from build123d import *

# Parameters (mm, degrees)
SKETCH_1_W      = 88
SKETCH_1_H      = 80
SKETCH_1_R      = 3
EXTRUDE_1_DEPTH = 3


with BuildPart() as part:
    # 草图1 → 凸台-拉伸1 (new body)
    with BuildSketch(Plane.XY):
        with Locations((-6, 0)):
            Rectangle(SKETCH_1_W, SKETCH_1_H)
        with Locations((-27, 25)):
            Circle(SKETCH_1_R, mode=Mode.SUBTRACT)
        with Locations(Location((27, 25, 0), (0, 0, 180))):
            Circle(SKETCH_1_R, mode=Mode.SUBTRACT)
        with Locations((27, -25)):
            Circle(SKETCH_1_R, mode=Mode.SUBTRACT)
        with Locations(Location((-27, -25, 0), (0, 0, 180))):
            Circle(SKETCH_1_R, mode=Mode.SUBTRACT)
        with Locations(Location((0, 0, 0), (0, 0, 180))):
            Circle(SKETCH_1_R, mode=Mode.SUBTRACT)
        with Locations(Location((-39, 0, 0), (0, 0, 180))):
            Circle(SKETCH_1_R, mode=Mode.SUBTRACT)
        with Locations(Location((-27, 0, 0), (0, 0, 180))):
            Circle(SKETCH_1_R, mode=Mode.SUBTRACT)
    extrude(amount=EXTRUDE_1_DEPTH)


solid = part.part
For this review, take the finished solid that the model builds, in its own axes (mm). Give positions to 0.01 mm unless a question says otherwise; leave off trailing zeros. Loops run counter-clockwise (first coordinate to the right, second up) from the corner with the lowest first, then second, coordinate; pieces in that order, holes last. Notation, with made-up numbers: M 17,-29 L 59,-29 A21 ccw 59,-8 Z; hole C 46.25,22.25 d4. An arc over 180 degrees is marked long. Answer as a JSON object with one key per item and string values. Group by question number.
Q1. Add section B-B on x = -39. Give the boundary of the cut face in (y, z), and give its area (3 significant figures).
Q2. For probe 1 along Y at (x, z) = (-27, 1.2); probe 2 along Y at (x, z) = (27, 1.75); probe 3 along Y at (x, z) = (0, 1.45), list the stretches that pass through material, from the lowest coordinate up. Write a range as [from, to].
Q3. Add section A-A on y = -25. Give the boundary of the cut face in (x, z), and give its area (3 significant figures).
Q4. Insertion check: P1, Ø5.5, axis at x = 27, y = 25, coming from the -Z side. The pin has a flat end and moves straight along its axis. Give the tip position at first contact, or say it passes through.
Q5. Add section C-C on z = 1.95. Give the boundary of the cut face in (x, y), and give its area (3 significant figures).
Q6. Mouldability with a two-part tool opening along X and no side actions: class faces 1 (the flat face through (-50, -1, 1)), 2 (the flat face through (38, -1, 1)), 3 (the flat face through (-7, 1, 3)), 4 (the cylindrical face through (24, -25, 1)) as +X half, -X half, draft (parallel to the pull), parting line (faces both ways), or undercut.
Q7. Add section D-D on x = -26. Give the boundary of the cut face in (y, z).
Checked values:
{
 "1": {"outline": "M -40,0 L -3,0 L -3,3 L -40,3 Z; M 3,0 L 40,0 L 40,3 L 3,3 Z", "area": "222 mm²"},
 "2": {"probe 1": "[-40, -28], [-22, -3], [3, 22], [28, 40]", "probe 2": "[-40, -28], [-22, 22], [28, 40]", "probe 3": "[-40, -3], [3, 40]"},
 "3": {"outline": "M -50,0 L -30,0 L -30,3 L -50,3 Z; M -24,0 L 24,0 L 24,3 L -24,3 Z; M 30,0 L 38,0 L 38,3 L 30,3 Z", "area": "228 mm²"},
 "4": {"P1": "through"},
 "5": {"outline": "M -50,-40 L 38,-40 L 38,40 L -50,40 Z; hole C -39,0 d6; hole C -27,-25 d6; hole C -27,0 d6; hole C -27,25 d6; hole C 0,0 d6; hole C 27,-25 d6; hole C 27,25 d6", "area": "6,840 mm²"},
 "6": {"face 1": "-X half", "face 2": "+X half", "face 3": "draft", "face 4": "undercut"},
 "7": {"outline": "M -40,0 L -27.83,0 L -27.83,3 L -40,3 Z; M -22.17,0 L -2.83,0 L -2.83,3 L -22.17,3 Z; M 2.83,0 L 22.17,0 L 22.17,3 L 2.83,3 Z; M 27.83,0 L 40,0 L 40,3 L 27.83,3 Z"}
}
